Input: part model. Units: mm. Frame: model coordinates. Coordinates: 2 decimals unless noted, no trailing zeros. Order: outer loops, then holes, each group sorted by start corner. A loop starts at its lowest first (then second) coordinate and runs counter-clockwise, first axis right, second up. Notation, with made-up numbers: (47, 63.5) - (96, 63.5) arc R5 cw to (96, 72.5) - close; hole circle Ø6 at (73, -29.75). An arc over 180 degrees is marked (long way). One line per question, with ' | ' between items.
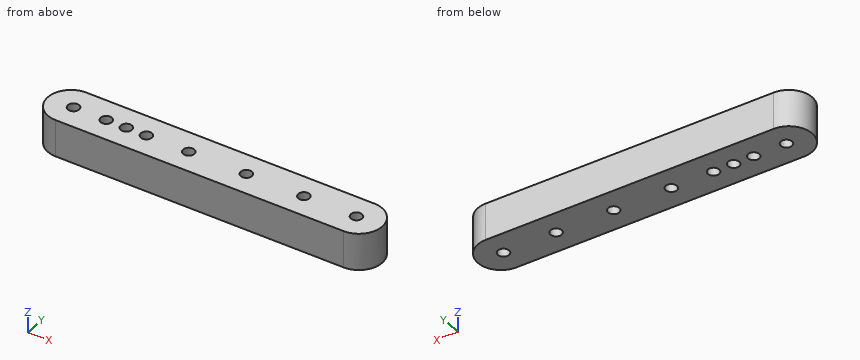
from build123d import *

# Parameters (mm, degrees)
BOSS_EXTRUDE1_DEPTH      = 2.8
BOSS_EXTRUDE1_DEPTH_BACK = 2.8
ECHELLE1_SCALE           = 2
SKETCH2_R                = 1.7
CUT_EXTRUDE6_DEPTH       = 11.2


with BuildPart() as part:
    # Sketch1 → Boss-Extrude1 (new, two sides: drawn at the far end of the back side and taken through both)
    with BuildSketch(Plane.XY.offset(-BOSS_EXTRUDE1_DEPTH_BACK)):
        with BuildLine():
            Line((-33.309608541, 3.5), (9.690391459, 3.5))
            ThreePointArc((9.690391459, 3.5), (13.190391459, 0), (9.690391459, -3.5))
            Line((9.690391459, -3.5), (-33.309608541, -3.5))
            ThreePointArc((-33.309608541, -3.5), (-36.809608541, 0), (-33.309608541, 3.5))
        make_face()
    extrude(amount=BOSS_EXTRUDE1_DEPTH + BOSS_EXTRUDE1_DEPTH_BACK)


with BuildPart() as part_1:
    # Echelle1: scaled about (-11.809608541, 0, 0)
    add(part.part.scale(ECHELLE1_SCALE).moved(Location((11.809608541, 0, 0))))

    # Sketch2 → Cut-Extrude6 (cut)
    with BuildSketch(Plane.XY.offset(-5.6)):
        with Locations((-38.289608541, 0)):
            Circle(SKETCH2_R)
        with Locations((-54.059608541, 0)):
            Circle(SKETCH2_R)
        with Locations((-19.659608541, 0)):
            Circle(SKETCH2_R)
        with Locations((-2.459608541, 0)):
            Circle(SKETCH2_R)
        with Locations((14.740391459, 0)):
            Circle(SKETCH2_R)
        with Locations((-44.289608541, 0)):
            Circle(SKETCH2_R)
        with Locations((-32.289608541, 0)):
            Circle(SKETCH2_R)
        with Locations((30.440391459, 0)):
            Circle(SKETCH2_R)
    extrude(amount=CUT_EXTRUDE6_DEPTH, mode=Mode.SUBTRACT)


solid = part_1.part
Item 1: Section A-A on z = -1.5. Count the separate pieces of the cut face and the enclosed holes in it, and give its area (3 significant figures).
Data:
separate pieces: 1 | enclosed holes: 8 | area: 1,290 mm^2
Item 2: Ray query, line 1 (Y direction, x = -43, z = 0.5); line 2 (X direction, y = -5.25, z = 3.75); line 3 (X direction, y = -2.5, z = -0.5). Return the intervals inside material, ascending.
Data:
line 1: -7 to -1.11, 1.11 to 7 | line 2: -59.44 to 35.82 | line 3: -61.35 to 37.73
Item 3: Section C-C on y = 3.75. Return the cut outline in (x, z), and give its area (3 significant figures).
Data:
outline: (-60.72, -5.6) - (37.1, -5.6) - (37.1, 5.6) - (-60.72, 5.6) - close | area: 1,100 mm^2
